Autodesk Inventor part; units mm, degrees
ref_plane "YZ Plane" through (0, 0, 0) normal (1, 0, 0) x (0, 1, 0)
ref_plane "XZ Plane" through (0, 0, 0) normal (0, 1, 0) x (-1, 0, 0)
ref_plane "XY Plane" through (0, 0, 0) normal (0, 0, 1) x (1, 0, 0)
sketch "草图1" plane through (0, 0, 0) normal (0, 0, 1) x (1, 0, 0)
  circle A0 centre (0, 0) radius 10
  dimension "d0" = 20
extrude "拉伸1" add sketch "草图1" along normal blind 108.34
sketch "草图2" plane through (0, 0, 108.34) normal (0, 0, 1) x (1, 0, 0)
  circle A0 centre (0, 0) radius 12.5
  dimension "d3" = 25
extrude "拉伸2" add sketch "草图2" against normal blind 0.6
sketch "草图3" plane through (0, 0, 0) normal (0, 1, 0) x (-1, 0, 0)
  line L0 (15.328, 4) -> (9.175, 4)
  line L1 (9.175, 4) -> (9.175, 5.2)
  line L2 (9.175, 5.2) -> (15.328, 5.2)
  line L3 (15.328, 5.2) -> (15.328, 4)
  line L4 (0, 0) -> (0, -10.7224)
  line L5 (-10, 0) -> (10, 0)
  dimension "d6" = 10.7224
  dimension "d7" = 1.2
  dimension "d8" = 4
  dimension "d9" = 9.175
  dimension "d10" = 6.153
revolve "旋转1" cut sketch "草图3" angle 360 about axis through (0, 0, 0) along (0, 0, -1)
chamfer "倒角1" distance 0.5 angle 45 1 edges at (-10, 0, 0)
properties part number "皮带轮轴"
The listing builds one solid part. Answer for the finished solid, in the listing's coordinates (mm). A direction names the side the tool comes from. Round coordinates to 2 decimals unless told otherwise and drop trailing zeros. Write each loop counter-clockwise with the first axis right and the second up, starting at its lowest first coordinate (ties: lowest second). Pieces come first, ordered by that corner, then holes. Notation, with made-up numbers: M 51.5,-29.75 L 67.5,-29.75 A24 ccw 67.5,-9.75 Z; hole C -10,-14 d11. An arc over 180 degrees is marked long. Write each question's results on one line, items separated by ' | '. Start each with the question number.
Item 1: For a pull along Z with two mould halves and no side action, classify faces 1 (the face through (-2.17, 9.76, 55.75)), 2 (the face through (-8.75, -2.76, 4.61)), 3 (the face through (0, 0, 0)) as pulls with the +Z half, pulls with the -Z half, needs draft (parallel to the pull), parting line crosses it, or undercut.
Item 2: For faces 4 (the face through (-9, -3, 5.2)), 5 (the face through (11.923, 3.755, 108.044)), 6 (the face through (-2.17, 9.76, 2.23)), determine the directions among +Z, -Z, +X, -X, +Y, -Y from which every point of the face is accessible in a straight line to the end or side of a thin tool.
Item 3: A cutting plane is placed at C-C on z = 73. Write down the section's boundary in (x, y), and give its area (3 significant figures).
Item 4: Flat-ended cylindrical pins translate along their axes: pin 1 Ø1.5 at (x, z) = (-4.5, 44.5) entering from +Y; pin 2 Ø3 at (x, z) = (1, 86) entering from -Y; pin 3 Ø6 at (y, z) = (-5.5, 12) entering from -X. Find the tip coordinate at first contact, or state that the pin passes through.
Item 5: Straight lines are drawn through the part: L1, parallel to Z at x = -10, y = -6.75; L2, parallel to Y at x = -0.25, z = 10; L3, parallel to X at y = 7, z = 96. For each, find the intervals that lie inside material, in ascending order. Write a range as [from, to].
Item 6: A cutting plane is placed at A-A on y = 0. Write down the section's boundary in (x, z) (3 decimals), and give its area (3 significant figures).
Check sheet entries:
1) face 1: needs draft | face 2: undercut | face 3: pulls with the -Z half
2) face 4: none | face 5: +Z, -Z | face 6: -Z
3) outline: C 0,0 d20 | area: 314 mm²
4) pin 1: y = 9.27 | pin 2: y = -10 | pin 3: x = -9.68
5) L1: [107.74, 108.34] | L2: [-10, 10] | L3: [-7.14, 7.14]
6) outline: M -12.5,107.74 L -10,107.74 L -10,5.2 L -9.175,5.2 L -9.175,4 L -10,4 L -10,0.5 L -9.5,0 L 9.5,0 L 10,0.5 L 10,4 L 9.175,4 L 9.175,5.2 L 10,5.2 L 10,107.74 L 12.5,107.74 L 12.5,108.34 L -12.5,108.34 Z | area: 2,170 mm²
